Autodesk Inventor part; units mm, degrees
ref_plane "YZ Plane" through (0, 0, 0) normal (1, 0, 0) x (0, 1, 0)
ref_plane "XZ Plane" through (0, 0, 0) normal (0, 1, 0) x (-1, 0, 0)
ref_plane "XY Plane" through (0, 0, 0) normal (0, 0, 1) x (1, 0, 0)
sketch "Sketch1" plane through (0, 0, 0) normal (0, 1, 0) x (-1, 0, 0)
  circle A0 centre (0, 0) radius 15
  circle A1 centre (0, 0) radius 7.5
  circle A2 centre (0, 7.5) radius 1.5
  circle A3 centre (0, -7.5) radius 1.5
  circle A4 centre (7.5, 0) radius 1.5
  circle A5 centre (-7.5, 0) radius 1.5
  dimension "d0" = 30
  dimension "d1" = 15
  dimension "d2" = 3
  dimension "d3" = 3
  dimension "d4" = 3
  dimension "d5" = 3
extrude "Extrusion1" add sketch "Sketch1" along normal blind 3 contours A0 | A4 A1 A3 A5 A2
properties part number "gearwheel_small"
Geometry check sheet. Reference: the model listing, model coordinates, mm. Coordinates: 2 decimals unless noted, no trailing zeros. Order: outer loops, then holes, each group sorted by start corner. A loop starts at its lowest first (then second) coordinate and runs counter-clockwise, first axis right, second up. Notation, with made-up numbers: (8, 69.5) -> (16, 69.5) arc R17 ccw to (16, 95.5) -> close; hole circle Ø9 at (-4, 13.5). An arc over 180 degrees is marked (long way). Use a Markdown table: item, result. Add a question column.
1. Cross-section at D-D (z = -7.5). Enter the section's corners in (x, y).
2. Mould release check, pull along X, two halves, no side actions. Record for faces 1 (the face through (14.985, 1.479, -0.66)), 2 (the face through (0, 0, 0)), 3 (the face through (0, 1, 9)): pulls with the +X half, pulls with the -X half, needs draft (parallel to the pull), parting line crosses it, or undercut.
3. Material ranges on L1, parallel to Z at x = 0, y = 1.1; L2, parallel to Z at x = -6.25, y = 2.6; L3, parallel to X at y = 1.8, z = 7, recorded low to high.
4. Cross-section at C-C (y = 2.4). Enter the section's corners in (x, z).
5. Cross-section at A-A (z = 0). Enter the section's corners in (x, y).
6. Go/stop test with a flat-tipped pin: pin 1 Ø1.5 at (x, y) = (-12, 2) entering from +Z. Record where the tip stops, or that it passes through.
7. Cross-section at B-B (x = -1). Enter the section's corners in (y, z).
Filled sheet:
| question | item | result |
|---|---|---|
| 1 | outline | (-12.99, 0) -> (-1.5, 0) -> (-1.5, 3) -> (-12.99, 3) -> close; (1.5, 0) -> (12.99, 0) -> (12.99, 3) -> (1.5, 3) -> close |
| 2 | face 1 | parting line crosses it |
| 2 | face 2 | needs draft |
| 2 | face 3 | undercut |
| 3 | L1 | -15 to -9, -6 to 6, 9 to 15 |
| 3 | L2 | -13.64 to -0.83, 0.83 to 13.64 |
| 3 | L3 | -13.27 to -1.41, 1.41 to 13.27 |
| 4 | outline | circle Ø30 at (0, 0); hole circle Ø3 at (-7.5, 0); hole circle Ø3 at (0, -7.5); hole circle Ø3 at (0, 7.5); hole circle Ø3 at (7.5, 0) |
| 5 | outline | (-15, 0) -> (-9, 0) -> (-9, 3) -> (-15, 3) -> close; (-6, 0) -> (6, 0) -> (6, 3) -> (-6, 3) -> close; (9, 0) -> (15, 0) -> (15, 3) -> (9, 3) -> close |
| 6 | pin 1 | z = 9.92 |
| 7 | outline | (0, -14.97) -> (3, -14.97) -> (3, -8.62) -> (0, -8.62) -> close; (0, -6.38) -> (3, -6.38) -> (3, 6.38) -> (0, 6.38) -> close; (0, 8.62) -> (3, 8.62) -> (3, 14.97) -> (0, 14.97) -> close |
